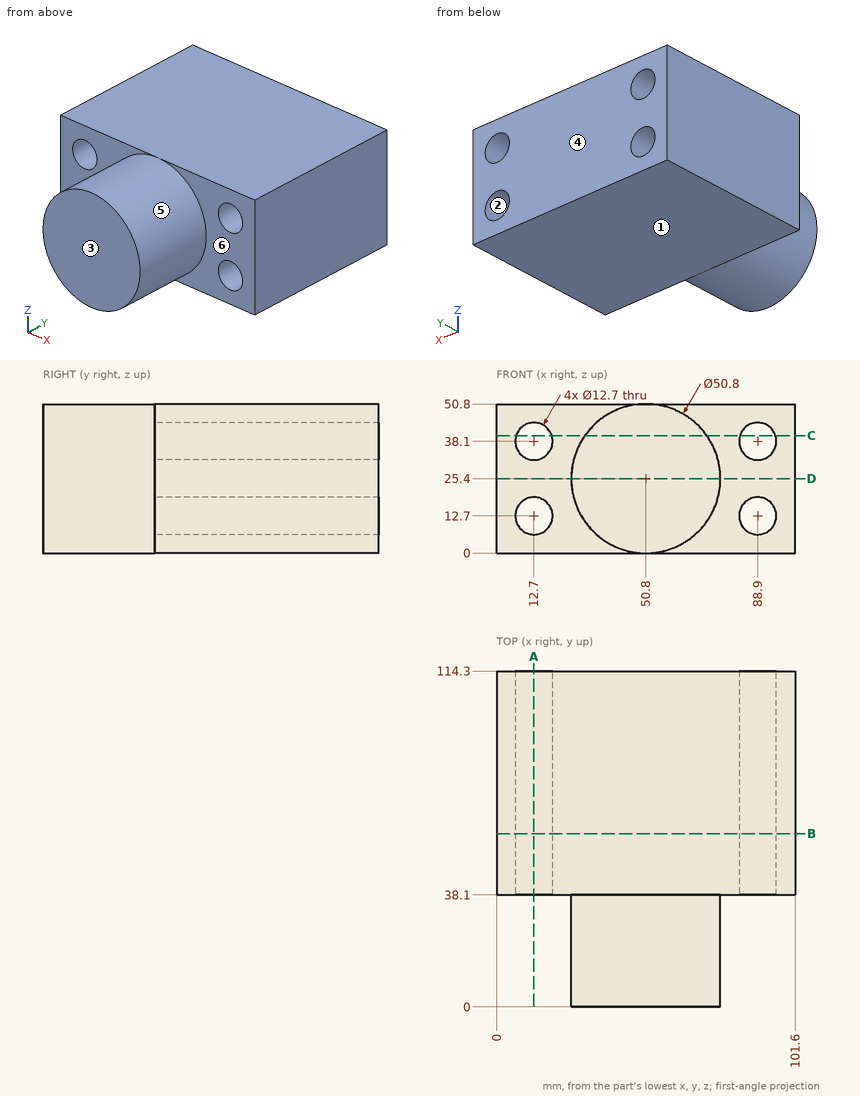
For this review, use the dimensioned drawing (mm, ordinates from the lowest corner) and the shaded views. A direction names the side the tool comes from. Give positions to 0.01 mm unless a question says otherwise; leave off trailing zeros. Order: outer loops, then holes, each group sorted by start corner. A loop starts at its lowest first (then second) coordinate and runs counter-clockwise, first axis right, second up.
1. Add section B-B, the plane y = 59. State the section outline as (x, z) points, then the cut area to 3 significant figures.
Solution:
outline: (0, 0) - (101.6, 0) - (101.6, 50.8) - (0, 50.8) - close; hole circle Ø12.7 at (12.7, 12.7); hole circle Ø12.7 at (12.7, 38.1); hole circle Ø12.7 at (88.9, 12.7); hole circle Ø12.7 at (88.9, 38.1)
area: 4,650 mm2
2. To check wall thickness, follow L1, parallel to Z at x = 88.9, y = 68.5; L2, parallel to X at y = 91, z = 38; L3, parallel to X at y = 90, z = 7.5. State the ranges of each line that lie inside material, in increasing order.
Solution:
L1: z = 0 to 6.35, 19.05 to 31.75, 44.45 to 50.8
L2: x = 0 to 6.35, 19.05 to 82.55, 95.25 to 101.6
L3: x = 0 to 9.06, 16.34 to 85.26, 92.54 to 101.6
3. Add section D-D, the plane z = 25.4. State the section outline as (x, y) points, then the cut area to 3 significant figures.
Solution:
outline: (0, 38.1) - (25.4, 38.1) - (25.4, 0) - (76.2, 0) - (76.2, 38.1) - (101.6, 38.1) - (101.6, 114.3) - (0, 114.3) - close
area: 9,680 mm2
4. Tool access review of the marked faces 4, 5 and 6: name each direction out of +Z, -Z, +X, -X, +Y, -Y from which nothing blocks a thin tool from reaching the whole face with its end or side.
Solution:
face 4: +Z, -Z, +X, -X, +Y
face 5: -Y
face 6: +X, -Y
5. Add section A-A, the plane x = 12.7. State the section outline as (y, z) points.
Solution:
outline: (38.1, 0) - (114.3, 0) - (114.3, 6.35) - (38.1, 6.35) - close; (38.1, 19.05) - (114.3, 19.05) - (114.3, 31.75) - (38.1, 31.75) - close; (38.1, 44.45) - (114.3, 44.45) - (114.3, 50.8) - (38.1, 50.8) - close
6. Add section C-C, the plane z = 40. State the section outline as (x, y) points, then the cut area to 3 significant figures.
Solution:
outline: (0, 38.1) - (6.64, 38.1) - (6.64, 114.3) - (0, 114.3) - close; (18.76, 38.1) - (30.02, 38.1) - (30.02, 0) - (71.58, 0) - (71.58, 38.1) - (82.84, 38.1) - (82.84, 114.3) - (18.76, 114.3) - close; (94.96, 38.1) - (101.6, 38.1) - (101.6, 114.3) - (94.96, 114.3) - close
area: 7,480 mm2
7. Mouldability with a two-part tool opening along Z and no side actions: class the marked faces 1, 2 and 3 as +Z half, -Z half, draft (parallel to the pull), parting line (faces both ways), or undercut.
Solution:
face 1: -Z half
face 2: undercut
face 3: draft
8. For pin 1 Ø2 at (x, y) = (40, 29) entering from -Z; pin 2 Ø11.5 at (x, z) = (88.9, 12.7) entering from +Y; pin 3 Ø20.5 at (x, z) = (12.7, 38.1) entering from -Y; pin 4 Ø3 at (y, z) = (29, 32.5) entering from +X (3 decimals), all flat-tipped, find the tip position at first contact; note any pin that passes through.
Solution:
pin 1: stops at z = 1.97
pin 2: passes through
pin 3: stops at y = 38.1
pin 4: stops at x = 75.575
